```python
from build123d import *

# Parameters (mm, degrees)
SKETCH2_R           = 1.5
SKETCH2_W           = 3
SKETCH2_H           = 6
SKETCH2_W_2         = 22
SKETCH2_H_2         = 22
BOSS_EXTRUDE2_DEPTH = 2.6


with BuildPart() as part:
    # Sketch2 → Boss-Extrude2 (new body)
    with BuildSketch(Plane(origin=(0, 0, 0), x_dir=(1, 0, 0), z_dir=(0, 1, 0))):
        with BuildLine():
            Line((-80, 45), (-80, 0))
            Line((-80, 0), (-65, 0))
            Line((-65, 0), (-65, -76))
            Line((-65, -76), (-73.74957627, -76))
            ThreePointArc((-73.74957627, -76), (0, -125), (73.74957627, -76))
            Line((73.74957627, -76), (65, -76))
            Line((65, -76), (65, 0))
            Line((65, 0), (80, 0))
            Line((80, 0), (80, 45))
            ThreePointArc((80, 45), (0, 125), (-80, 45))
        make_face()
        with Locations(Location((-42, -99, 0), (0, 0, 270))):
            Circle(SKETCH2_R, mode=Mode.SUBTRACT)
        with Locations((-62.5, -56)):
            Rectangle(SKETCH2_W, SKETCH2_H, mode=Mode.SUBTRACT)
        with Locations((-40.5, -56)):
            Rectangle(SKETCH2_W, SKETCH2_H, mode=Mode.SUBTRACT)
        with Locations((-31, -38)):
            Rectangle(SKETCH2_W_2, SKETCH2_H_2, mode=Mode.SUBTRACT)
        with Locations(Location((42, -99, 0), (0, 0, 270))):
            Circle(SKETCH2_R, mode=Mode.SUBTRACT)
        with Locations((40.5, -56)):
            Rectangle(SKETCH2_W, SKETCH2_H, mode=Mode.SUBTRACT)
        with Locations((31, -38)):
            Rectangle(SKETCH2_W_2, SKETCH2_H_2, mode=Mode.SUBTRACT)
        with Locations((62.5, -56)):
            Rectangle(SKETCH2_W, SKETCH2_H, mode=Mode.SUBTRACT)
        with Locations(Location((-14, 95.5, 0), (0, 0, 270))):
            Circle(SKETCH2_R, mode=Mode.SUBTRACT)
        with Locations(Location((-14, 117.5, 0), (0, 0, 270))):
            Circle(SKETCH2_R, mode=Mode.SUBTRACT)
        with Locations(Location((14, 95.5, 0), (0, 0, 270))):
            Circle(SKETCH2_R, mode=Mode.SUBTRACT)
        with Locations(Location((14, 117.5, 0), (0, 0, 270))):
            Circle(SKETCH2_R, mode=Mode.SUBTRACT)
    extrude(amount=BOSS_EXTRUDE2_DEPTH)


solid = part.part
```
Design review of the part built by this model. Coordinates are the model's own, in mm. Coordinates: 2 decimals unless noted, no trailing zeros. Order: outer loops, then holes, each group sorted by start corner. A loop starts at its lowest first (then second) coordinate and runs counter-clockwise, first axis right, second up.
1) Wall thickness on line 1 along X through (y, z) = (1.3, 57); line 2 along X through (y, z) = (0.7, 45.5); line 3 along X through (y, z) = (1.1, 99): over which ranges is each line inside the solid? List them lowest first.
2) Take a section at C-C, the plane x = 51. Give the boundary of the cut face in (y, z).
3) Take a section at A-A, the plane y = 2.2. State how many separate pieces and enclosed holes the cut face has, and give its area (3 significant figures).
4) Clearance check with flat-ended pins moving along their axes: pin 1 (1.3 mm diameter, centred on y = 1.5, z = 54.5, fed in from +X); pin 2 (1.3 mm diameter, centred on y = 1.5, z = 39.5, fed in from -X); pin 3 (1.3 mm diameter, centred on x = -68.5, y = 1.5, fed in from -Z). State where each tip first meets the part, or that it passes through.
5) Take a section at B-B, the plane z = 66. Give the boundary of the cut face in (x, y), and give its area (3 significant figures).
Returned:
1. line 1: x = -65 to -64, -61 to -42, -39 to 39, 42 to 61, 64 to 65
1. line 2: x = -65 to -42, -20 to 20, 42 to 65
1. line 3: x = -59.03 to -43.5, -40.5 to 40.5, 43.5 to 59.03
2. outline: (0, -106.64) - (2.6, -106.64) - (2.6, 106.64) - (0, 106.64) - close
3. separate pieces: 1
3. enclosed holes: 12
3. area: 31,300 mm2
4. pin 1: stops at x = 65
4. pin 2: stops at x = -65
4. pin 3: stops at z = -87.38
5. outline: (-65, 0) - (65, 0) - (65, 2.6) - (-65, 2.6) - close
5. area: 338 mm2
